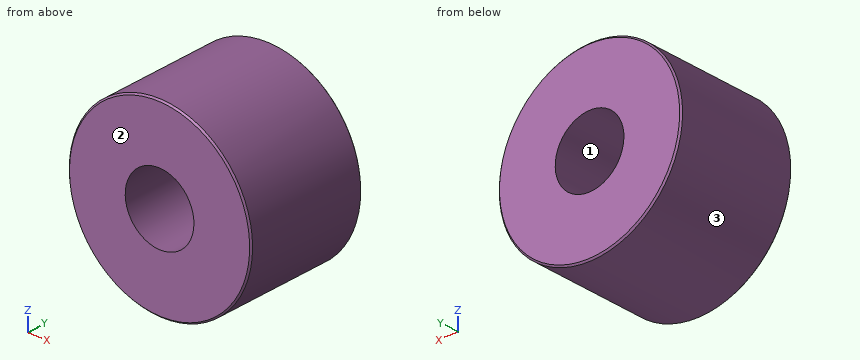
Autodesk Inventor part; units mm, degrees
ref_plane "YZ Plane" through (0, 0, 0) normal (1, 0, 0) x (0, 1, 0)
ref_plane "XZ Plane" through (0, 0, 0) normal (0, 1, 0) x (-1, 0, 0)
ref_plane "XY Plane" through (0, 0, 0) normal (0, 0, 1) x (1, 0, 0)
sketch "Sketch1" plane through (0, 0, 0) normal (0, 1, 0) x (-1, 0, 0)
  circle A0 centre (0, 0) radius 6
  dimension "d0" = 12
extrude "Extrusion1" add sketch "Sketch1" against normal blind 8
chamfer "Chamfer1" distance 0.1 angle 45 2 edges at (6, -8, 0) (6, 0, 0)
sketch "Sketch2" plane through (0, -8, 0) normal (0, -1, 0) x (1, 0, 0)
  point P0 (0, 0)
hole "Hole1" at (0, -8, 0) direction (0, 1, 0) diameter 4.5 end through all
properties part number "13-0004" material "Polystyrene, High Impact"
Design review of the part built by this model. Coordinates are the model's own, in mm. Face numbers are marked on the shaded views. Coordinates: 2 decimals unless noted, no trailing zeros. Write each loop counter-clockwise with the first axis right and the second up, starting at its lowest first coordinate (ties: lowest second). Pieces come first, ordered by that corner, then holes. Notation, with made-up numbers: (7, 76.5) - (32, 76.5) arc R22 cw to (32, 100.5) - close; hole circle Ø10 at (60, -7.75). An arc over 180 degrees is marked (long way). One line per item, written item: value.
1) Add section A-A (z = 0). State the section outline as (x, y) points, plus the area to 3 significant figures.
Answer sheet:
outline: (-6, -7.9) - (-5.9, -8) - (-2.25, -8) - (-2.25, 0) - (-5.9, 0) - (-6, -0.1) - close; (2.25, -8) - (5.9, -8) - (6, -7.9) - (6, -0.1) - (5.9, 0) - (2.25, 0) - close
area: 60.0 mm2
2) Insertion check: pin 1 (2 mm diameter, centred on x = -3.5, y = -6, fed in from +Z). The pin has a flat end and moves straight along its axis. Give the tip position at first contact, or say it passes through.
Answer sheet:
pin 1: stops at z = 5.45
3) Add section B-B (y = -3.5). State the section outline as (x, z) points, plus the area to 3 significant figures.
Answer sheet:
outline: circle Ø12 at (0, 0); hole circle Ø4.5 at (0, 0)
area: 97.2 mm2
4) Mouldability with a two-part tool opening along X and no side actions: class the marked faces 1, 2 and 3 as +X half, -X half, draft (parallel to the pull), parting line (faces both ways), or undercut.
Answer sheet:
face 1: undercut
face 2: draft
face 3: parting line
5) To check wall thickness, follow probe 1 along Z at (x, y) = (0, -3); probe 2 along Z at (x, y) = (-0.75, -4.5); probe 3 along X at (y, z) = (-7.5, -1.5). State the ranges of each line that lie inside material, in increasing order.
Answer sheet:
probe 1: z = -6 to -2.25, 2.25 to 6
probe 2: z = -5.95 to -2.12, 2.12 to 5.95
probe 3: x = -5.81 to -1.68, 1.68 to 5.81
